```python
from build123d import *

# Parameters (mm, degrees)
F0_W      = 60
F0_H      = 60
F1_DEPTH  = 10
F2_W      = 60
F2_H      = 60
F3_DEPTH  = 25
F5_DEPTH  = 51.5
F7_DEPTH  = 10
F8_W      = 19.9074504152
F8_H      = 1.7359393835
F8_W_2    = 45
F8_W_3    = 24.514567852
F9_DEPTH  = 10
F10_W     = 2.977065742
F10_H     = 29.9195116386
F11_DEPTH = 10


with BuildPart() as f1:
    # F0 (on Top) → F1 (new body)
    with BuildSketch(Plane.XY):
        Rectangle(F0_W, F0_H)
    extrude(amount=F1_DEPTH)

    # F2 (on face) → F3 (join)
    with BuildSketch(Plane.XY.offset(10)):
        Rectangle(F2_W, F2_H)
        with Locations((60, 0)):
            Rectangle(F2_W, F2_H)
    extrude(amount=F3_DEPTH)

    # F4 (on face) → F5 (cut)
    with BuildSketch(Plane.XY.offset(35)):
        with BuildLine():
            ThreePointArc((60, 0), (57.0710678119, 7.0710678119), (50, 10))
            ThreePointArc((50, 10), (42.9289321881, -7.0710678119), (60, 0))
        make_face()
        with BuildLine():
            ThreePointArc((15, 0), (12.0710678119, 7.0710678119), (5, 10))
            ThreePointArc((5, 10), (-2.0710678119, -7.0710678119), (15, 0))
        make_face()
    extrude(amount=-F5_DEPTH, mode=Mode.SUBTRACT)

    # F6 (on face) → F7 (cut)
    with BuildSketch(Plane.XY.offset(35)):
        Polygon((5, 29.9537748588), (-15.0160359405, 29.9537740648), (-15.0160359405, -30), (74.7204658659, -30), (74.7204658659, -15.0462223754), (89.7204658659, -15.0462223754), (89.7204658659, 14.9537776246), (74.7204658659, 14.9537776246), (74.7204658659, 29.9537776246), (50, 29.953776644), align=None)
        with BuildLine():
            ThreePointArc((15, 0), (-2.0710678119, -7.0710678119), (5, 10))
            ThreePointArc((5, 10), (12.0710678119, 7.0710678119), (15, 0))
        make_face(mode=Mode.SUBTRACT)
        with BuildLine():
            ThreePointArc((60, 0), (42.9289321881, -7.0710678119), (50, 10))
            ThreePointArc((50, 10), (57.0710678119, 7.0710678119), (60, 0))
        make_face(mode=Mode.SUBTRACT)
    extrude(amount=-F7_DEPTH, mode=Mode.SUBTRACT)

    # F8 (on face) → F9 (cut)
    with BuildSketch(Plane.XY.offset(35)):
        with Locations((-4.9537252076, 29.1320303082)):
            Rectangle(F8_W, F8_H)
        with Locations((27.5, 29.1320303082)):
            Rectangle(F8_W_2, F8_H)
        with Locations((62.257283926, 29.1320303082)):
            Rectangle(F8_W_3, F8_H)
    extrude(amount=-F9_DEPTH, mode=Mode.SUBTRACT)

    # F10 (on face) → F11 (cut)
    with BuildSketch(Plane.XY.offset(35)):
        with Locations((91.1140106618, -0.0397800468)):
            Rectangle(F10_W, F10_H)
    extrude(amount=-F11_DEPTH, mode=Mode.SUBTRACT)


solid = f1.part
```
For this review, take the finished solid that the model builds, in its own axes (mm). A direction names the side the tool comes from. Coordinates: 2 decimals unless noted, no trailing zeros. Loops run counter-clockwise (first coordinate to the right, second up) from the corner with the lowest first, then second, coordinate; pieces in that order, holes last. Notation, with made-up numbers: (-15.75, -1) - (43.25, -1) arc R19 cw to (43.25, 7) - close; hole circle Ø2 at (-31, 70.25). An arc over 180 degrees is marked (long way). Use one line per item in the form item = value. Start each with the question number.
1) To check wall thickness, follow probe 1 along X at (y, z) = (0, 14); probe 2 along X at (y, z) = (15, 29); probe 3 along X at (y, z) = (0, 7.25). State the ranges of each line that lie inside material, in increasing order. Write a range as from..to.
2) Take a section at B-B (z = 12). State the section outline as (x, y) points.
3) Draft analysis for pull direction X (two halves, no side actions). For faces 1 (the face through (74.72, -23, 30)), 2 (the face through (-30, 0, 17)), state which applies: released by +X, released by -X, zero draft, split by the parting line, or undercut.
4) For pin 1 (18 mm diameter, centred on x = 71.5, y = -15, fed in from -Z); pin 2 (4 mm diameter, centred on x = 50, y = 18, fed in from +Z); pin 3 (8 mm diameter, centred on y = -4.5, z = 5.5, fed in from +X), all flat-tipped, find the tip position at first contact; note any pin that passes through.
5) Take a section at D-D (y = 20). State the section outline as (x, z) points.
6) Take a section at C-C (x = 47.5). State the section outline as (y, z) points, plus the area to 3 significant figures.
7) Take a section at A-A (y = -8). State the section outline as (x, z) points, plus the area to 3 significant figures.
8) For faces 3 (the face through (66, 0, 10)), 4 (the face through (-15.016, 0, 30)), list the 3-axis set-ups (+Z, -Z, +X, -X, +Y, -Y) from which the entire face can be reached by the end or side of a thin tool; tool diameter is ignored.
From the geometry:
q1.probe_1 = -30..-5, 15..40, 60..90
q1.probe_2 = -30..-15.02, 74.72..90
q1.probe_3 = -30..-5, 15..30
q2.outline = (-30, -30) - (90, -30) - (90, 30) - (-30, 30) - close; hole circle Ø20 at (5, 0); hole circle Ø20 at (50, 0)
q3.face_1 = undercut
q3.face_2 = released by -X
q4.pin_1 = 10
q4.pin_2 = 25
q4.pin_3 = 30
q5.outline = (-30, 0) - (30, 0) - (30, 10) - (90, 10) - (90, 35) - (74.72, 35) - (74.72, 25) - (-15.02, 25) - (-15.02, 35) - (-30, 35) - close
q6.outline = (-30, 10) - (-9.68, 10) - (-9.68, 25) - (-30, 25) - close; (9.68, 10) - (30, 10) - (30, 25) - (9.68, 25) - close
q6.area = 610 mm2
q7.outline = (-30, 0) - (-1, 0) - (-1, 25) - (-15.02, 25) - (-15.02, 35) - (-30, 35) - close; (11, 0) - (30, 0) - (30, 10) - (44, 10) - (44, 25) - (11, 25) - close; (56, 10) - (90, 10) - (90, 25) - (56, 25) - close
q7.area = 2,070 mm2
q8.face_3 = -Z, +X, +Y, -Y
q8.face_4 = +Z, -Y
